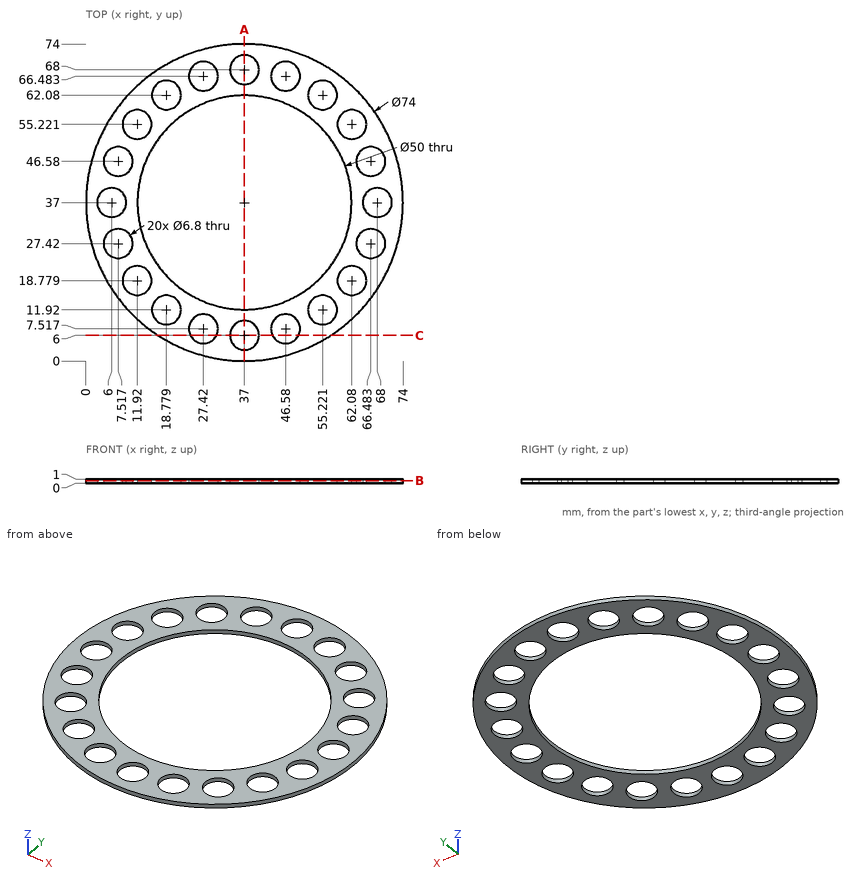
Geometry check sheet. Reference: drawing and pictorial views, mm from the part's lowest x, y, z. Give positions to 0.01 mm unless a question says otherwise; leave off trailing zeros. Write each loop counter-clockwise with the first axis right and the second up, starting at its lowest first coordinate (ties: lowest second). Pieces come first, ordered by that corner, then holes. Notation, with made-up numbers: (35.25, 74) -> (50.25, 74) arc R15 ccw to (50.25, 102) -> close; hole circle Ø2 at (7.5, 25). An arc over 180 degrees is marked (long way). One line per item, written item: value. Start each with the question number.
Item 1: Section check C-C on y = 6. Record the cut outline in (x, z).
Item 2: Section check A-A on x = 37. Record the cut outline in (y, z), then the cut area to 3 significant figures.
Item 3: Material ranges on probe 1 along Y at (x, z) = (37, 0.6); probe 2 along X at (y, z) = (64, 0.85) (1 decimal); probe 3 along X at (y, z) = (56.5, 0.1) (1 decimal), recorded low to high. Write a range as from..to.
Item 4: Section check B-B on z = 0.6. State how many separate pieces and enclosed holes the cut face has, then the cut area to 3 significant figures.
Results list:
1. outline: (16.8, 0) -> (24.38, 0) -> (24.38, 1) -> (16.8, 1) -> close; (30.46, 0) -> (33.6, 0) -> (33.6, 1) -> (30.46, 1) -> close; (40.4, 0) -> (43.54, 0) -> (43.54, 1) -> (40.4, 1) -> close; (49.62, 0) -> (57.2, 0) -> (57.2, 1) -> (49.62, 1) -> close
2. outline: (0, 0) -> (2.6, 0) -> (2.6, 1) -> (0, 1) -> close; (9.4, 0) -> (12, 0) -> (12, 1) -> (9.4, 1) -> close; (62, 0) -> (64.6, 0) -> (64.6, 1) -> (62, 1) -> close; (71.4, 0) -> (74, 0) -> (74, 1) -> (71.4, 1) -> close
2. area: 10.4 mm²
3. probe 1: 0..2.6, 9.4..12, 62..64.6, 71.4..74
3. probe 2: 11.7..16, 21.6..25.1, 29.7..44.3, 48.9..52.4, 58..62.3
3. probe 3: 5.6..8.8, 15.1..21.4, 52.6..58.9, 65.2..68.4
4. separate pieces: 1
4. enclosed holes: 21
4. area: 1,610 mm²
